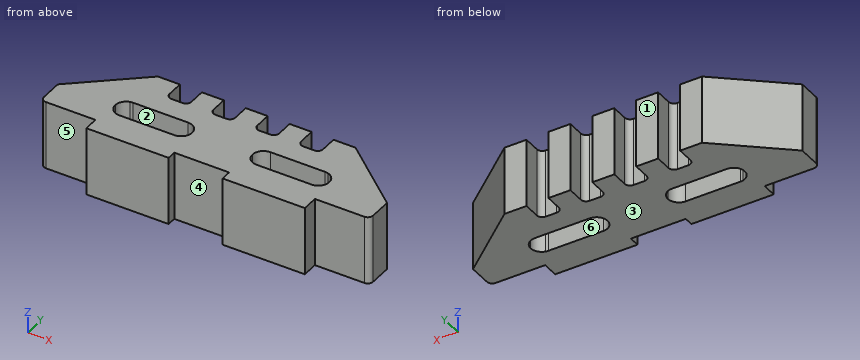
```python
from build123d import *

# Parameters (mm, degrees)
F1_DEPTH = 25


with BuildPart() as f1:
    # F0 (on Top) → F1 (new body)
    with BuildSketch(Plane.XY):
        with BuildLine():
            Line((-75, 17.161901), (-75, 33.278717))
            Line((-75, 33.278717), (-99, 13.278717))
            Line((-99, 13.278717), (-99, 5.278717))
            ThreePointArc((-99, 5.278717), (-98.414214, 3.864503), (-97, 3.278717))
            Line((-97, 3.278717), (-79, 3.278717))
            Line((-79, 3.278717), (-79, -1.999241))
            Line((-79, -1.999241), (-75, -1.999241))
            Line((-75, -1.999241), (-75, 9.395945))
            ThreePointArc((-75, 9.395945), (-77.202197, 10.829057), (-78.040169, 13.319295))
            Line((-78.040169, 13.319295), (-78.040164, 13.319706))
            ThreePointArc((-78.040164, 13.319706), (-77.177183, 15.760739), (-75, 17.161901))
        make_face()
        with BuildLine():
            Line((-67, 33.278717), (-75, 33.278717))
            Line((-75, 33.278717), (-75, 17.161901))
            ThreePointArc((-75, 17.161901), (-74.523729, 17.249405), (-74.040374, 17.278717))
            Line((-74.040374, 17.278717), (-54, 17.278717))
            ThreePointArc((-54, 17.278717), (-51.171718, 16.107289), (-50, 13.279128))
            Line((-50, 13.279128), (-50, 13.278717))
            ThreePointArc((-50, 13.278717), (-51.171718, 10.450556), (-54, 9.279128))
            Line((-54, 9.279128), (-74.04037, 9.279128))
            ThreePointArc((-74.04037, 9.279128), (-74.523727, 9.30844), (-75, 9.395945))
            Line((-75, 9.395945), (-75, -1.999241))
            Line((-75, -1.999241), (-49, -1.999241))
            Line((-49, -1.999241), (-49, 1.278717))
            Line((-49, 1.278717), (-39, 1.278717))
            Line((-39, 1.278717), (-29, 1.278717))
            Line((-29, 1.278717), (-29, -2.541677))
            Line((-29, -2.541677), (-2.966445, -2.541677))
            Line((-2.966445, -2.541677), (-2.966445, 9.414552))
            ThreePointArc((-2.966445, 9.414552), (-3.478779, 9.312821), (-4, 9.278717))
            Line((-4, 9.278717), (-24, 9.278717))
            ThreePointArc((-24, 9.278717), (-26.828427, 10.450289), (-28, 13.278717))
            ThreePointArc((-28, 13.278717), (-26.828427, 16.107144), (-24, 17.278717))
            Line((-24, 17.278717), (-4, 17.278717))
            ThreePointArc((-4, 17.278717), (-3.478779, 17.244612), (-2.966445, 17.142881))
            Line((-2.966445, 17.142881), (-2.966445, 33.278717))
            Line((-2.966445, 33.278717), (-11, 33.278717))
            Line((-11, 33.278717), (-11, 27.278717))
            ThreePointArc((-11, 27.278717), (-11.585786, 25.864503), (-13, 25.278717))
            Line((-13, 25.278717), (-17, 25.278717))
            ThreePointArc((-17, 25.278717), (-18.414214, 25.864503), (-19, 27.278717))
            Line((-19, 27.278717), (-19, 33.278717))
            Line((-19, 33.278717), (-27, 33.278717))
            Line((-27, 33.278717), (-27, 27.278717))
            ThreePointArc((-27, 27.278717), (-27.585786, 25.864503), (-29, 25.278717))
            Line((-29, 25.278717), (-33, 25.278717))
            ThreePointArc((-33, 25.278717), (-34.414214, 25.864503), (-35, 27.278717))
            Line((-35, 27.278717), (-35, 33.278717))
            Line((-35, 33.278717), (-43, 33.278717))
            Line((-43, 33.278717), (-43, 27.278717))
            ThreePointArc((-43, 27.278717), (-43.585786, 25.864503), (-45, 25.278717))
            Line((-45, 25.278717), (-49, 25.278717))
            ThreePointArc((-49, 25.278717), (-50.414214, 25.864503), (-51, 27.278717))
            Line((-51, 27.278717), (-51, 33.278717))
            Line((-51, 33.278717), (-59, 33.278717))
            Line((-59, 33.278717), (-59, 27.278717))
            ThreePointArc((-59, 27.278717), (-59.585786, 25.864503), (-61, 25.278717))
            Line((-61, 25.278717), (-65, 25.278717))
            ThreePointArc((-65, 25.278717), (-66.414214, 25.864503), (-67, 27.278717))
            Line((-67, 27.278717), (-67, 33.278717))
        make_face()
        with BuildLine():
            Line((-2.966445, 9.414552), (-2.966445, -2.541677))
            Line((-2.966445, -2.541677), (1, -2.541677))
            Line((1, -2.541677), (1, 3.278773))
            Line((1, 3.278773), (19.0067, 3.278773))
            ThreePointArc((19.0067, 3.278773), (20.418539, 3.862189), (21.006688, 5.272062))
            Line((21.006688, 5.272062), (21.033555, 13.278717))
            Line((21.033555, 13.278717), (-2.966445, 33.278717))
            Line((-2.966445, 33.278717), (-2.966445, 17.142881))
            ThreePointArc((-2.966445, 17.142881), (-0.827129, 15.714469), (0, 13.278717))
            ThreePointArc((0, 13.278717), (-0.827129, 10.842964), (-2.966445, 9.414552))
        make_face()
    extrude(amount=F1_DEPTH)


solid = f1.part
```
Verification items for the finished model (mm, model axes). Face numbers are marked on the shaded views. A direction names the side the tool comes from. Round coordinates to 2 decimals unless told otherwise and drop trailing zeros. Write each loop counter-clockwise with the first axis right and the second up, starting at its lowest first coordinate (ties: lowest second). Pieces come first, ordered by that corner, then holes.
1. Section check A-A on x = -70.5. Enter the section's corners in (y, z).
2. Section check C-C on x = 3.5. Enter the section's corners in (y, z), plus the area to 3 significant figures.
3. Draft check along Y on the marked faces 1, 2 and 3. Enter one of: +Y half, -Y half, draft (parallel to the pull), parting line (faces both ways), or undercut.
4. Section check D-D on y = 20.5. Enter the section's corners in (x, z).
5. Scan lines: L1, parallel to X at y = 1, z = 23.75; L2, parallel to Y at x = -9, z = 3; L3, parallel to X at y = 27, z = 7.25. Record each from-to range of solid material in increasing order.
6. Section check B-B on z = 8.5. State how many separate pieces and enclosed holes the cut face has, plus the area to 3 significant figures.
7. Gauge pin test, flat ends, axial feed: P1, Ø4, axis at y = 0, z = 11, coming from the -X side; P2, Ø1.2, axis at x = -31, z = 17.5, coming from the +Y side; P3, Ø1, axis at y = -0.5, z = 14, coming from the +X side; P4, Ø3, axis at x = -26, y = 27.5, coming from the -Z side. Record the tip position at first contact, or that the pin passes through.
8. Access from +Z, -Z, +X, -X, +Y, -Y to the whole of each face (thin tool, end or side, straight path). Record for the marked faces 4, 5 and 6.
Answer:
1. outline: (-2, 0) - (9.28, 0) - (9.28, 25) - (-2, 25) - close; (17.28, 0) - (33.28, 0) - (33.28, 25) - (17.28, 25) - close
2. outline: (3.28, 0) - (27.89, 0) - (27.89, 25) - (3.28, 25) - close
2. area: 615 mm2
3. face 1: +Y half
3. face 2: undercut
3. face 3: draft
4. outline: (-90.33, 0) - (12.37, 0) - (12.37, 25) - (-90.33, 25) - close
5. L1: x = -79 to -49, -29 to 1
5. L2: y = -2.54 to 9.28, 17.28 to 33.28
5. L3: x = -82.53 to -66.98, -59.02 to -50.98, -43.02 to -34.98, -27.02 to -18.98, -11.02 to 4.57
6. separate pieces: 1
6. enclosed holes: 2
6. area: 2,820 mm2
7. P1: stops at x = -79
7. P2: stops at y = 25.28
7. P3: stops at x = 1
7. P4: stops at z = 0
8. face 4: +Z, -Z, -Y
8. face 5: +Z, -Z, -X, -Y
8. face 6: +Z, -Z
